Part model, mm, in its own coordinate system. A direction names the side the tool comes from. Coordinates: 2 decimals unless noted, no trailing zeros. Write each loop counter-clockwise with the first axis right and the second up, starting at its lowest first coordinate (ties: lowest second). Pieces come first, ordered by that corner, then holes. Notation, with made-up numbers: (-26, 70.5) -> (24, 70.5) arc R16 cw to (24, 95.5) -> close; hole circle Ø9 at (16.5, 28.5). An arc over 180 degrees is marked (long way). One line per question, with ' | ' between items. Start each with the question number.
Item 1: Saw through at C-C (y = 2). List the corners of the cut face in (x, z).
Item 2: Two-plate mould, pull along Z, no slides. Class faces 5 (the flat face through (-3.4, 10.39, -0.38)), 6 (the cylindrical face through (6.88, 6.04, 6.77)), 7 (the flat face through (4, 8, -11)): pulls with the +Z half, pulls with the -Z half, needs draft (parallel to the pull), parting line crosses it, or undercut.
Item 3: Probe probe 1 along Z at (x, y) = (7, 9.75); probe 2 along X at (y, z) = (7.5, 0.25); probe 3 along X at (y, z) = (2.5, -3.5). List the from-to ranges inside material, lowest first. Write a range as [from, to].
Item 4: Pin check, flat tips, straight feed: pin 1 (1.1 mm diameter, centred on x = -4.5, z = -3.5, fed in from -Y); pin 2 (5 mm diameter, centred on x = 9, y = 5, fed in from -Z); pin 3 (1 mm diameter, centred on x = -3, y = 3, fed in from -Z); pin 4 (4 mm diameter, centred on x = 10.5, z = 2, fed in from +Y). Stop position of each tip, or through.
Item 5: Saw through at B-B (z = -0.25). Count the separate pieces of the cut face and the enclosed holes in it, and give its area (3 significant figures).
Item 6: Saw through at A-A (y = 6). List the corners of the cut face in (x, z).
Item 7: Saw through at D-D (y = 7.75). List the corners of the cut face in (x, z).
Item 8: 3-axis set-ups, long thin cutter, end or side, ignore diameter. For faces 1 (the flat face through (4, 0, -3)), 2 (the flat face through (4, 4, -11)), 3 (the flat face through (13, 5, -3)), 4 (the flat face through (11.15, 10.41, -0.36)): which of +Z, -Z, +X, -X, +Y, -Y reach the whole face in a straight line?
from build123d import *

# Parameters (mm, degrees)
SKETCH_1_R               = 10
EXTRUDE_1_DEPTH          = 12
CUT_EXTRUDE_1_DEPTH      = 23.353389068
SKETCH_3_R               = 8
CUT_EXTRUDE_2_DEPTH      = 11
FILLET_1_R               = 3
CUT_EXTRUDE_3_DEPTH      = 23.353389241
CUT_EXTRUDE_3_DEPTH_BACK = 23.353389241
SKETCH_5_W               = 1.508883289
SKETCH_5_H               = 1
SKETCH_5_H_2             = 0.980176719
SKETCH_5_W_2             = 1.789126732
EXTRUDE_3_DEPTH          = 2.5
CHAMFER_2_SIZE           = 0.8


with BuildPart() as part:
    # 草图1 → 凸台-拉伸1 (new body)
    with BuildSketch(Plane(origin=(0, 0, 0), x_dir=(1, 0, 0), z_dir=(0, 1, 0))):
        with Locations(Location((3.877687805, 2.770426149, 0), (0, 0, 270))):
            Circle(SKETCH_1_R)
    extrude(amount=EXTRUDE_1_DEPTH)

    # 草图2 → 切除-拉伸1 (cut, through all)
    with BuildSketch(Plane.XY):
        with BuildLine():
            Line((0.877687805, 8), (6.877687805, 8))
            ThreePointArc((6.877687805, 8), (8.877687805, 6), (6.877687805, 4))
            Line((6.877687805, 4), (0.877687805, 4))
            ThreePointArc((0.877687805, 4), (-1.122312195, 6), (0.877687805, 8))
        make_face()
    extrude(amount=-CUT_EXTRUDE_1_DEPTH, mode=Mode.SUBTRACT)

    # 草图3 → 切除-拉伸2 (cut)
    with BuildSketch(Plane(origin=(0, 12, 0), x_dir=(1, 0, 0), z_dir=(0, 1, 0))):
        with Locations(Location((3.877687805, 2.770426149, 0), (0, 0, 270))):
            Circle(SKETCH_3_R)
    extrude(amount=-CUT_EXTRUDE_2_DEPTH, mode=Mode.SUBTRACT)

    # 圆角1
    # the kernel refuses this fillet: 3 mm, written as the material it adds along each edge
    with BuildSketch(Plane(origin=(3.877687805, 1, -2.770426149), x_dir=(0, 0, 1), z_dir=(-1, 0, 0))) as fillet_1_piece_1:
        with BuildLine():
            CenterArc((8 - FILLET_1_R, FILLET_1_R), FILLET_1_R, 270, 90)
            Line((8 - FILLET_1_R, 0), (8, 0))
            Line((8, 0), (8, FILLET_1_R))
        make_face()
    revolve(axis=Axis((3.877687805, 1, -2.770426149), (0, 1, 0)))
    # the kernel refuses this fillet: 3 mm, written as the material it takes off along each edge
    with BuildSketch(Plane(origin=(3.877687805, 0, -2.770426149), x_dir=(0, 0, 1), z_dir=(-1, 0, 0))) as fillet_1_2_piece_1:
        with BuildLine():
            CenterArc((10 - FILLET_1_R, FILLET_1_R), FILLET_1_R, 270, 90)
            Line((10 - FILLET_1_R, 0), (10, 0))
            Line((10, 0), (10, FILLET_1_R))
        make_face()
    revolve(axis=Axis((3.877687805, 0, -2.770426149), (0, 1, 0)), mode=Mode.SUBTRACT)
    with BuildSketch(Plane(origin=(3.877687805, 12, -2.770426149), x_dir=(0, 0, 1), z_dir=(-1, 0, 0))) as fillet_1_2_piece_2:
        with BuildLine():
            CenterArc((7, -2.828427125), FILLET_1_R, 0, 70.528779366)
            Line((8, 0), (10, 0))
            Line((10, 0), (10, -2.828427125))
        make_face()
    revolve(axis=Axis((3.877687805, 12, -2.770426149), (0, 1, 0)), mode=Mode.SUBTRACT)

    # 草图4 → 切除-拉伸3 (cut, two sides: drawn at the far end of the back side and taken through both)
    with BuildSketch(Plane(origin=(0, 0, 0), x_dir=(0, 0, -1), z_dir=(1, 0, 0)).offset(-CUT_EXTRUDE_3_DEPTH_BACK)):
        with BuildLine():
            Line((0.770426149, 7), (4.770426149, 7))
            ThreePointArc((4.770426149, 7), (5.770426149, 6), (4.770426149, 5))
            Line((4.770426149, 5), (0.770426149, 5))
            ThreePointArc((0.770426149, 5), (-0.229573851, 6), (0.770426149, 7))
        make_face()
    extrude(amount=CUT_EXTRUDE_3_DEPTH + CUT_EXTRUDE_3_DEPTH_BACK, mode=Mode.SUBTRACT)

    # 草图5 → 凸台-拉伸3 (add)
    with BuildSketch(Plane(origin=(0, 10.8, 0), x_dir=(-1, 0, 0), z_dir=(0, -1, 0))):
        with Locations((-11.601062589, 5.270426149)):
            Rectangle(SKETCH_5_W, SKETCH_5_H)
        with Locations((-11.601062589, 0.280337789)):
            Rectangle(SKETCH_5_W, SKETCH_5_H_2)
        with Locations((3.999711661, 5.270426149)):
            Rectangle(SKETCH_5_W_2, SKETCH_5_H)
        with Locations((3.999711661, 0.270426149)):
            Rectangle(SKETCH_5_W_2, SKETCH_5_H)
    extrude(amount=EXTRUDE_3_DEPTH)

    # 倒角2
    chamfer_2_edges = [part.edges().sort_by_distance(p)[0] for p in [
        (11.235137721, 10.8, -0.770426149),
        (-3.486713591, 10.8, -4.770426149),
        (-3.486713591, 10.8, -0.770426149),
        (11.235137721, 10.8, -4.770426149),
    ]]
    chamfer(chamfer_2_edges, length=CHAMFER_2_SIZE)


solid = part.part
From the geometry:
1) outline: circle Ø19.66 at (3.88, -2.77); hole circle Ø14.47 at (3.88, -2.77)
2) face 5: undercut | face 6: parting line crosses it | face 7: needs draft
3) probe 1: [-12.21, -10.14], [4.6, 6.67] | probe 2: [-5.66, -3.53], [11.29, 13.41] | probe 3: [-6.05, -3.69], [11.44, 13.81]
4) pin 1: y = 0.13 | pin 2: z = -12.36 | pin 3: z = -10.47 | pin 4: y = 12
5) separate pieces: 3 | enclosed holes: 0 | area: 57.8 mm2
6) outline: (-5.66, -5.77) arc R10 ccw to (-1.12, -11.43) -> (-1.12, -9.02) arc R8 cw to (-3.54, -5.77) -> close; (-5.66, 0.23) -> (-3.54, 0.23) arc R8 cw to (11.29, 0.23) -> (13.42, 0.23) arc R10 ccw to start; (8.88, -11.43) arc R10 ccw to (13.42, -5.77) -> (11.29, -5.77) arc R8 cw to (8.88, -9.02) -> close
7) outline: (-0.09, -11.95) -> (-0.09, -9.72) arc R8 cw (long way) to (7.85, -9.72) -> (7.85, -11.95) arc R10 ccw (long way) to start
8) face 1: +Z, -Z, +X, -X, -Y | face 2: -Z | face 3: +X, -X | face 4: +Y
